Can you work these out from the model? Positions are in its coordinate system, mm. A direction names the side the tool comes from. Coordinates: 2 decimals unless noted, no trailing zeros. Write each loop counter-clockwise with the first axis right and the second up, starting at its lowest first coordinate (ties: lowest second). Pieces come first, ordered by that corner, then holes. Notation, with made-up numbers: (15, 15.5) -> (23, 15.5) arc R27 cw to (23, 49.5) -> close; hole circle Ø1 at (65.25, -21.75). An arc over 180 degrees is marked (long way). Use one line per item in the form item = value.
Autodesk Inventor part; units mm, degrees
ref_plane "YZ Plane" through (0, 0, 0) normal (1, 0, 0) x (0, 1, 0)
ref_plane "XZ Plane" through (0, 0, 0) normal (0, 1, 0) x (-1, 0, 0)
ref_plane "XY Plane" through (0, 0, 0) normal (0, 0, 1) x (1, 0, 0)
sketch "Sketch1" plane through (0, 0, 0) normal (0, 0, 1) x (1, 0, 0)
  line L0 (13.335, -13.335) -> (-13.335, -13.335) construction
  line L1 (-13.335, -13.335) -> (-13.335, 13.335)
  line L2 (-13.335, 13.335) -> (13.335, 13.335)
  line L3 (13.335, 13.335) -> (13.335, -13.335)
  line L4 (13.335, -13.335) -> (-13.335, 13.335) construction
  line L5 (-13.335, -13.335) -> (13.335, 13.335) construction
  line L6 (18.415, 18.415) -> (-18.415, 18.415)
  line L7 (-18.415, 18.415) -> (-18.415, -18.415)
  line L8 (-18.415, -18.415) -> (18.415, -18.415)
  line L9 (18.415, -18.415) -> (18.415, 18.415)
  line L10 (-13.335, -13.335) -> (-13.335, -18.415)
  line L11 (13.335, -13.335) -> (13.335, -18.415)
  point P0 (0, 0)
  dimension "d0" = 26.67
  dimension "d1" = 26.67
  dimension "d2" = 5.08
extrude "Extrusion1" add sketch "Sketch1" along normal blind 12.7 contours L10 L8 L7 L6 L9 L11 L3 L2 L1
sketch "Sketch2" plane through (18.415, -18.415, 0) normal (1, 0, 0) x (0, 0, -1)
  line L0 (0, 0) -> (0, 36.83)
  line L1 (0, 36.83) -> (-12.7, 36.83)
  line L2 (-12.7, 0) -> (-12.7, 36.83)
  line L3 (0, 0) -> (-12.7, 0)
  line L4 (0, 36.83) -> (-12.7, 36.83) construction
  line L5 (-6.35, 36.83) -> (-6.35, 0) construction
  line L6 (0, 0) -> (-12.7, 0) construction
  line L7 (0, 31.75) -> (-12.7, 31.75) construction
  line L8 (-12.7, 0) -> (-12.7, 31.75) construction
  line L9 (-12.7, 15.875) -> (0, 15.875) construction
  line L10 (0, 0) -> (0, 31.75) construction
  circle A0 centre (-6.35, 15.875) radius 2.25
  circle A1 centre (-6.35, 15.875) radius 5.715
  point P0 (0, 18.415)
  dimension "d5" = 4.5
  dimension "d6" = 11.43
extrude "Extrusion2" cut sketch "Sketch2" against normal through all contours A0
extrude "Extrusion3" cut sketch "Sketch2" against normal blind 2.54 contours A1
sketch "Sketch3" plane through (-18.415, -18.415, 0) normal (-1, 0, 0) x (0, 0, 1)
  circle A0 centre (6.35, 15.875) radius 2.25
  circle A1 centre (6.35, 15.875) radius 5.715
  point P0 (0, 18.415)
  dimension "d11" = 11.43
extrude "Extrusion4" cut sketch "Sketch3" against normal blind 2.54
properties part number "Inner_Tube_Endcap2"
Q1. Thinking about a two-plate mould opening in Z: for faces 6 (the flat face through (-1, 14, 0)), 7 (the flat face through (15.875, -5, 6)), 8 (the flat face through (-16, -18.415, 6)), which applies, released by +Z, released by -Z, zero draft, split by the parting line, or undercut?
Return value:
face_6 = released by -Z
face_7 = undercut
face_8 = zero draft
Q2. Suppose I cut it at D-D (x = -14). Write out the boundary of the cut face in (y, z) (3 decimals), then the cut area to 3 significant figures.
Return value:
outline = (-18.415, 0) -> (18.415, 0) -> (18.415, 12.7) -> (-18.415, 12.7) -> close; hole circle Ø4.5 at (-2.54, 6.35)
area = 452 mm2
Q3. Suppose I cut it at A-A (z = 6.35). Write out the boundary of the cut face in (x, y) (3 decimals), then the cut area to 3 significant figures.
Return value:
outline = (-18.415, -18.415) -> (-13.335, -18.415) -> (-13.335, -4.79) -> (-15.875, -4.79) -> (-15.875, -8.255) -> (-18.415, -8.255) -> close; (-18.415, 3.175) -> (-15.875, 3.175) -> (-15.875, -0.29) -> (-13.335, -0.29) -> (-13.335, 13.335) -> (13.335, 13.335) -> (13.335, -0.29) -> (15.875, -0.29) -> (15.875, 3.175) -> (18.415, 3.175) -> (18.415, 18.415) -> (-18.415, 18.415) -> close; (13.335, -18.415) -> (18.415, -18.415) -> (18.415, -8.255) -> (15.875, -8.255) -> (15.875, -4.79) -> (13.335, -4.79) -> close
area = 429 mm2
Q4. If I drill on line 1 (X direction, y = -5.5, z = 12) (3 decimals); line 2 (X direction, y = 2, z = 5) (3 decimals); line 3 (Z direction, x = -14.4, y = -2.54), over which ranges is the centre line in solid material (lowest first)? Write a range as from..to.
Return value:
line_1 = -18.415..-13.335, 13.335..18.415
line_2 = -15.875..-13.335, 13.335..15.875
line_3 = 0..4.1, 8.6..12.7
Q5. Will these pins go through, and if not, where does the flat tip stop? pin 1 (5 mm diameter, centred on y = -2.54, z = 6.35, fed in from -X) (3 decimals); pin 2 (2 mm diameter, centred on x = -9, z = 1.5, fed in from -Y) (3 decimals); pin 3 (2.5 mm diameter, centred on y = -2.54, z = 6.35, fed in from +X); pin 4 (3 mm diameter, centred on x = -13.5, y = 0.5, fed in from -Z).
Return value:
pin_1 = -15.875
pin_2 = 13.335
pin_3 = through
pin_4 = 0
Q6. Suppose I cut it at B-B (y = -2.54). Write out the boundary of the cut face in (x, z) (3 decimals), then the cut area to 3 significant figures.
Return value:
outline = (-18.415, 0) -> (-13.335, 0) -> (-13.335, 4.1) -> (-15.875, 4.1) -> (-15.875, 0.635) -> (-18.415, 0.635) -> close; (-18.415, 12.065) -> (-15.875, 12.065) -> (-15.875, 8.6) -> (-13.335, 8.6) -> (-13.335, 12.7) -> (-18.415, 12.7) -> close; (13.335, 0) -> (18.415, 0) -> (18.415, 0.635) -> (15.875, 0.635) -> (15.875, 4.1) -> (13.335, 4.1) -> close; (13.335, 8.6) -> (15.875, 8.6) -> (15.875, 12.065) -> (18.415, 12.065) -> (18.415, 12.7) -> (13.335, 12.7) -> close
area = 48.1 mm2
Q7. Suppose I cut it at C-C (y = 9). Write out the boundary of the cut face in (x, z) (3 decimals), then the cut area to 3 significant figures.
Return value:
outline = (-18.415, 0) -> (-13.335, 0) -> (-13.335, 12.7) -> (-18.415, 12.7) -> close; (13.335, 0) -> (18.415, 0) -> (18.415, 12.7) -> (13.335, 12.7) -> close
area = 129 mm2
Q8. For faces 1 (the flat face through (-13.335, -2, 9)), 2 (the cylindrical face through (14.623, -1.864, 4.204)), 3 (the flat face through (16, -18.415, 6)), 4 (the cylindrical face through (17.163, 1.322, 10.562)), 5 (the cylindrical face through (-17.16, -4.73, 11.63)), which set-ups out of +Z, -Z, +X, -X, +Y, -Y let a thin tool reach every point of the face, with its end or its side?
Return value:
face_1 = +Z, -Z, -Y
face_2 = +X, -X
face_3 = +Z, -Z, +X, -X, -Y
face_4 = +X
face_5 = -X
